```python
from build123d import *

# Parameters (mm, degrees)
SKETCH1_R           = 15
SKETCH1_R_2         = 4
BOSS_EXTRUDE1_DEPTH = 5
SKETCH3_R           = 15
SKETCH3_R_2         = 11.1125
BOSS_EXTRUDE2_DEPTH = 80
BOSS_EXTRUDE3_START = -2
SKETCH4_R           = 11.1125
BOSS_EXTRUDE3_DEPTH = 2
SKETCH5_W           = 4
SKETCH5_H           = 6.16515139
BOSS_EXTRUDE4_DEPTH = 5
SKETCH6_W           = 10
SKETCH6_H           = 11.320508076
BOSS_EXTRUDE5_DEPTH = 5
SKETCH8_R           = 4
CUT_EXTRUDE1_DEPTH  = 4
SKETCH10_W          = 4
SKETCH10_H          = 6.16515139
CUT_EXTRUDE2_DEPTH  = 2
SKETCH11_W          = 10
SKETCH11_H          = 11.320508076
CUT_EXTRUDE3_DEPTH  = 18.5


with BuildPart() as part:
    # Sketch1 → Boss-Extrude1 (new body)
    with BuildSketch(Plane.XY):
        with BuildLine():
            Line((-16.301967128, -6.363636364), (-6.98655734, -30.227272727))
            ThreePointArc((-6.98655734, -30.227272727), (0, -35), (6.98655734, -30.227272727))
            Line((6.98655734, -30.227272727), (16.301967128, -6.363636364))
            ThreePointArc((16.301967128, -6.363636364), (17.5, 0), (16.301967128, 6.363636364))
            Line((16.301967128, 6.363636364), (6.98655734, 30.227272727))
            ThreePointArc((6.98655734, 30.227272727), (0, 35), (-6.98655734, 30.227272727))
            Line((-6.98655734, 30.227272727), (-16.301967128, 6.363636364))
            ThreePointArc((-16.301967128, 6.363636364), (-17.5, 0), (-16.301967128, -6.363636364))
        make_face()
        Circle(SKETCH1_R, mode=Mode.SUBTRACT)
        with Locations((0, 27.5)):
            Circle(SKETCH1_R_2, mode=Mode.SUBTRACT)
        with Locations((0, -27.5)):
            Circle(SKETCH1_R_2, mode=Mode.SUBTRACT)
    extrude(amount=BOSS_EXTRUDE1_DEPTH)

    # Sketch3 → Boss-Extrude2 (add)
    with BuildSketch(Plane.XY):
        Circle(SKETCH3_R)
        Circle(SKETCH3_R_2, mode=Mode.SUBTRACT)
    extrude(amount=BOSS_EXTRUDE2_DEPTH)

    # Sketch4 → Boss-Extrude3 (add)
    with BuildSketch(Plane.XY.offset(80).offset(BOSS_EXTRUDE3_START)):
        Circle(SKETCH4_R)
    extrude(amount=BOSS_EXTRUDE3_DEPTH)

    # Sketch5 → Boss-Extrude4 (add)
    with BuildSketch(Plane.XY.offset(80)):
        with BuildLine():
            Line((-2, 12.082575695), (2, 12.082575695))
            ThreePointArc((2, 12.082575695), (5, 7.5), (2, 2.917424305))
            Line((2, 2.917424305), (-2, 2.917424305))
            ThreePointArc((-2, 2.917424305), (-5, 7.5), (-2, 12.082575695))
        make_face()
        with Locations((0, 7.5)):
            Rectangle(SKETCH5_W, SKETCH5_H, mode=Mode.SUBTRACT)
    extrude(amount=BOSS_EXTRUDE4_DEPTH)

    # Sketch6 → Boss-Extrude5 (add)
    with BuildSketch(Plane(origin=(0, 12.5, 0), x_dir=(1, 0, 0), z_dir=(0, 1, 0))):
        with BuildLine():
            Line((-5, -28.339745962), (5, -28.339745962))
            ThreePointArc((5, -28.339745962), (10, -37), (5, -45.660254038))
            Line((5, -45.660254038), (-5, -45.660254038))
            ThreePointArc((-5, -45.660254038), (-10, -37), (-5, -28.339745962))
        make_face()
        with Locations((0, -37)):
            Rectangle(SKETCH6_W, SKETCH6_H, mode=Mode.SUBTRACT)
    extrude(amount=BOSS_EXTRUDE5_DEPTH)

    # Sketch7 → Revolve1 (revolve)
    with BuildSketch(Plane(origin=(0, 0, 0), x_dir=(0, 0, -1), z_dir=(1, 0, 0))):
        Polygon((0, 15), (4, 12.690598923), (4, 0), (0, 0), align=None)
    revolve(axis=Axis((0, 0, -4), (0, 0, 1)))

    # Sketch8 → Cut-Extrude1 (cut)
    with BuildSketch(Plane(origin=(0, 0, -4), x_dir=(-1, 0, 0), z_dir=(0, 0, -1))):
        with Locations(Location((0, 0, 0), (0, 0, 90))):
            Circle(SKETCH8_R)
    extrude(amount=-CUT_EXTRUDE1_DEPTH, mode=Mode.SUBTRACT)

    # Sketch10 → Cut-Extrude2 (cut)
    with BuildSketch(Plane.XY.offset(80)):
        with Locations((0, 7.5)):
            Rectangle(SKETCH10_W, SKETCH10_H)
    extrude(amount=-CUT_EXTRUDE2_DEPTH, mode=Mode.SUBTRACT)

    # Sketch11 → Cut-Extrude3 (cut, symmetric)
    with BuildSketch(Plane(origin=(0, 12.5, 0), x_dir=(1, 0, 0), z_dir=(0, 1, 0))):
        with Locations((0, -37)):
            Rectangle(SKETCH11_W, SKETCH11_H)
    extrude(amount=CUT_EXTRUDE3_DEPTH, both=True, mode=Mode.SUBTRACT)


solid = part.part
```
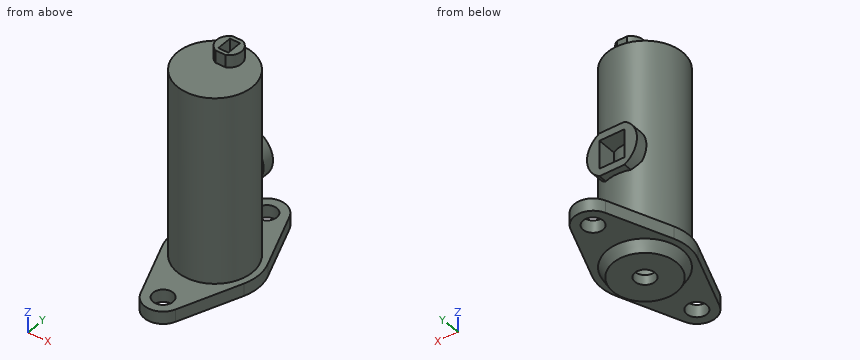
The model under review builds one solid part; all positions refer to its coordinate system, in mm. Round coordinates to 2 decimals unless told otherwise and drop trailing zeros. Write each loop counter-clockwise with the first axis right and the second up, starting at its lowest first coordinate (ties: lowest second). Pieces come first, ordered by that corner, then holes. Notation, with made-up numbers: (11, 21) - (30, 21) arc R8 ccw to (30, 33) - close; hole circle Ø9 at (37, -31.75). An arc over 180 degrees is marked (long way). Use one line per item in the form item = value.
Q1. Consider section A-A (z = 13.5). State the section outline as (x, y) points (1 decimal).
Answer key:
outline = circle Ø30 at (0, 0); hole circle Ø22.2 at (0, 0)
Q2. For line 1 (Z direction, x = 6, y = 3.5); line 2 (Z direction, x = -7, y = 18.5); line 3 (Y direction, x = -1.5, z = 56), list the stretches that pass through material, from the lowest coordinate up. Write a range as [from, to].
Answer key:
line_1 = [-4, 0], [78, 80]
line_2 = [0, 5]
line_3 = [-14.92, -11.01], [11.01, 14.92]
Q3. Consider section C-C (z = 34.5). State the section outline as (x, y) points (1 decimal).
Answer key:
outline = (-9.7, 12.5) - (-8.3, 12.5) arc R15 ccw (long way) to (8.3, 12.5) - (9.7, 12.5) - (9.7, 17.5) - (5, 17.5) - (5, 9.9) arc R11.1 cw (long way) to (-5, 9.9) - (-5, 17.5) - (-9.7, 17.5) - close
Q4. Insertion check: pin 1 Ø2 at (x, z) = (-0.5, 81.5) entering from +Y; pin 2 Ø1.9 at (x, z) = (9.5, 35.5) entering from -Y; pin 3 Ø9 at (x, y) = (-2, -4.5) entering from +Z; pin 4 Ø10.5 at (x, y) = (0, 0) entering from -Z. Each pin has a flat end and moves straight along its axis. Give the tip position at first contact, or say it passes through.
Answer key:
pin_1 = 12.08
pin_2 = -12.32
pin_3 = 80
pin_4 = -4
Q5. Consider section D-D (x = -3). State how many separate pieces and enclosed holes the cut face has, and give its area (3 significant figures).
Answer key:
separate_pieces = 4
enclosed_holes = 0
area = 925 mm2
Q6. Consider section B-B (y = 0). State the section outline as (x, z) points.
Answer key:
outline = (-17.5, 0) - (-15, 0) - (-12.69, -4) - (-4, -4) - (-4, 0) - (-11.11, 0) - (-11.11, 78) - (11.11, 78) - (11.11, 0) - (4, 0) - (4, -4) - (12.69, -4) - (15, 0) - (17.5, 0) - (17.5, 5) - (15, 5) - (15, 80) - (-15, 80) - (-15, 5) - (-17.5, 5) - close
